from build123d import *

# Parameters (mm, degrees)
SKETCH_1_W          = 180
SKETCH_1_H          = 50
EXTRUDE_1_DEPTH     = 30
SKETCH_2_W          = 40
SKETCH_2_H          = 50
EXTRUDE_2_DEPTH     = 80
FILLET_1_R          = 25
SKETCH_3_R          = 12.5
CUT_EXTRUDE_2_DEPTH = 145.913767462
SKETCH_7_W          = 25
SKETCH_7_H          = 50
EXTRUDE_5_DEPTH     = 80
EXTRUDE_6_REACH     = 213.019
SKETCH_9_W          = 65
SKETCH_9_H          = 330.441162185
CUT_EXTRUDE_4_DEPTH = 401.320460854
SKETCH_10_W         = 50
SKETCH_10_H         = 30
EXTRUDE_7_DEPTH     = 10
SKETCH_11_W         = 50
SKETCH_11_H         = 30
CUT_EXTRUDE_5_DEPTH = 5
SKETCH_12_R         = 7.5
CUT_EXTRUDE_6_DEPTH = 412.962042251


with BuildPart() as part:
    # 草图1 → 凸台-拉伸1 (new body)
    with BuildSketch(Plane(origin=(0, 0, 0), x_dir=(1, 0, 0), z_dir=(0, 1, 0))):
        with Locations((90, -25)):
            Rectangle(SKETCH_1_W, SKETCH_1_H)
    extrude(amount=EXTRUDE_1_DEPTH)

    # 草图2 → 凸台-拉伸2 (add)
    with BuildSketch(Plane.XZ):
        with Locations((90, 25)):
            Rectangle(SKETCH_2_W, SKETCH_2_H)
    extrude(amount=EXTRUDE_2_DEPTH)

    # 圆角1
    fillet_1_edges = [part.edges().sort_by_distance(p)[0] for p in [
        (90, -80, 50),
        (90, -80, 0),
    ]]
    fillet(fillet_1_edges, radius=FILLET_1_R - 0.0001)  # a hair under: the kernel refuses the full size

    # 草图3 → 切除-拉伸2 (cut, through all)
    with BuildSketch(Plane(origin=(110, 0, 0), x_dir=(0, 0, -1), z_dir=(1, 0, 0))):
        with Locations((-25, -55)):
            Circle(SKETCH_3_R)
    extrude(amount=-CUT_EXTRUDE_2_DEPTH, mode=Mode.SUBTRACT)

    # 草图7 → 凸台-拉伸5 (add)
    with BuildSketch(Plane(origin=(0, 30, 0), x_dir=(1, 0, 0), z_dir=(0, 1, 0))):
        with Locations((19.5, -25)):
            Rectangle(SKETCH_7_W, SKETCH_7_H)
        with Locations((160.5, -25)):
            Rectangle(SKETCH_7_W, SKETCH_7_H)
    extrude(amount=EXTRUDE_5_DEPTH)

    # 凸台-拉伸6: up to this face of the body (flat: up to its plane)
    extrude_6_end = Plane(part.part.faces().sort_by_distance((7, 70, 25))[0])
    # 草图8 → 凸台-拉伸6 (add, up to the picked face)
    with BuildSketch(Plane(origin=(173, 0, 0), x_dir=(0, 0, -1), z_dir=(1, 0, 0)), mode=Mode.PRIVATE) as extrude_6_sk1:
        with BuildLine():
            Line((0, 110), (-79.29372145, 110))
            add(Edge.make_bspline(
                [(-79.29372145, 110), (123.322725029, 174.375095478), (335.808448859, 110)],
                knots=[0, 0, 0, 1, 1, 1], degree=2))
            add(Edge.make_bspline(
                [(335.808448859, 110), (344.655163531, 85.008885119), (332.386652106, 65.024574676)],
                knots=[0, 0, 0, 1, 1, 1], degree=2))
            add(Edge.make_bspline(
                [(332.386652106, 65.024574676), (334.882025134, 94.793074398), (307.328252939, 102.88474179)],
                knots=[0, 0, 0, 1, 1, 1], degree=2))
            add(Edge.make_bspline(
                [(307.328252939, 102.88474179), (153.571097441, 138.708355764), (0, 110)],
                knots=[0, 0, 0, 1, 1, 1], degree=2))
        make_face()
    extrude_6_tool1 = split(extrude(extrude_6_sk1.sketch, amount=-EXTRUDE_6_REACH, mode=Mode.PRIVATE), bisect_by=extrude_6_end, keep=Keep.BOTH, mode=Mode.PRIVATE)
    add(extrude_6_tool1.solids().sort_by(Axis((173, 122.914419, -143.709252), (-1, 0, 0)))[0])

    # 草图9 → 切除-拉伸4 (cut, through all)
    with BuildSketch(Plane(origin=(0, 30, 0), x_dir=(1, 0, 0), z_dir=(0, 1, 0))):
        with Locations((90, 198.149530653)):
            Rectangle(SKETCH_9_W, SKETCH_9_H)
    extrude(amount=CUT_EXTRUDE_4_DEPTH, mode=Mode.SUBTRACT)

    # 草图10 → 凸台-拉伸7 (add)
    with BuildSketch(Plane(origin=(180, 0, 0), x_dir=(0, 0, -1), z_dir=(1, 0, 0))):
        with Locations((-25, 15)):
            Rectangle(SKETCH_10_W, SKETCH_10_H)
    extrude(amount=EXTRUDE_7_DEPTH)

    # 草图11 → 切除-拉伸5 (cut)
    with BuildSketch(Plane(origin=(190, 0, 0), x_dir=(0, 0, -1), z_dir=(1, 0, 0))):
        with Locations((-25, 15)):
            Rectangle(SKETCH_11_W, SKETCH_11_H)
    extrude(amount=-CUT_EXTRUDE_5_DEPTH, mode=Mode.SUBTRACT)

    # 草图12 → 切除-拉伸6 (cut, through all)
    with BuildSketch(Plane(origin=(185, 0, 0), x_dir=(0, 0, -1), z_dir=(1, 0, 0))):
        with Locations((-25, 15)):
            Circle(SKETCH_12_R)
    extrude(amount=-CUT_EXTRUDE_6_DEPTH, mode=Mode.SUBTRACT)


solid = part.part
Source: CAD feature listing. Evaluate the final solid. Frame: model axes, mm. A direction names the side the tool comes from. Round coordinates to 2 decimals unless told otherwise and drop trailing zeros. Loops run counter-clockwise (first coordinate to the right, second up) from the corner with the lowest first, then second, coordinate; pieces in that order, holes last.
Q1. Mould query, pull axis Z, two halves, no side actions, for faces 6 (the face through (90.28, -72.482, 42.871)), 7 (the face through (93.795, 15.33, 32.493)), 8 (the face through (32, 69, 25)), 9 (the face through (71, 26, 0)). Classes: pulls with the +Z half, pulls with the -Z half, needs draft (parallel to the pull), parting line crosses it, or undercut.
Q2. Section A-A, the plane y = 15. Return loops of the section in (x, z), plus the area to 4 significant figures.
Q3. Access query for faces 1 (the face through (71, 26, 50)), 2 (the face through (89, 30, 25)), 3 (the face through (179, 30, 25)), 4 (the face through (35, 0, 25)), 5 (the face through (7, 123, -83)). Directions: +Z, -Z, +X, -X, +Y, -Y. A direction counts if a zero-diameter tool reaches every point of the face in a straight line with its end or side. Return the directions, or none.
Q4. Section B-B, the plane x = 85.5. State how many separate pieces and enclosed holes the cut face has, plus the area to 3 significant figures.
Q5. First-contact query: P1, Ø8, axis at x = 54, y = 112.5, coming from the -Z side; P2, Ø3.5, axis at x = 2, z = 37.5, coming from the +Y side; P3, Ø25, axis at y = 65, z = 28.5, coming from the -X side. Flat tips, straight axial feed; report the tip coordinate or a pass-through.
Q6. Ray query, line 1 (X direction, y = 126.5, z = -74); line 2 (Y direction, x = 40.5, z = 25); line 3 (Y direction, x = 91.5, z = 25). Return the intervals inside material, ascending.
Solutions:
1. face 6: pulls with the +Z half
1. face 7: undercut
1. face 8: needs draft
1. face 9: undercut
2. outline: (0, 0) - (185, 0) - (185, 17.5) - (0, 17.5) - close; (0, 32.5) - (185, 32.5) - (185, 50) - (0, 50) - close
2. area: 6,475 mm2
3. face 1: +Z, +X, -X, -Y
3. face 2: +Z, -Z
3. face 3: +Z, -Z, +X, +Y
3. face 4: +Z, -Z, -X, -Y
3. face 5: +Z, -Z, -X, +Y
4. separate pieces: 2
4. enclosed holes: 2
4. area: 6,100 mm2
5. P1: stops at z = -336.32
5. P2: stops at y = 30
5. P3: stops at x = 7
6. line 1: x = 7 to 57.5, 122.5 to 173
6. line 2: y = 0 to 7.5, 22.5 to 30, 110 to 124.9
6. line 3: y = -80 to -67.5, -42.5 to 7.5, 22.5 to 30, 110 to 124.9
